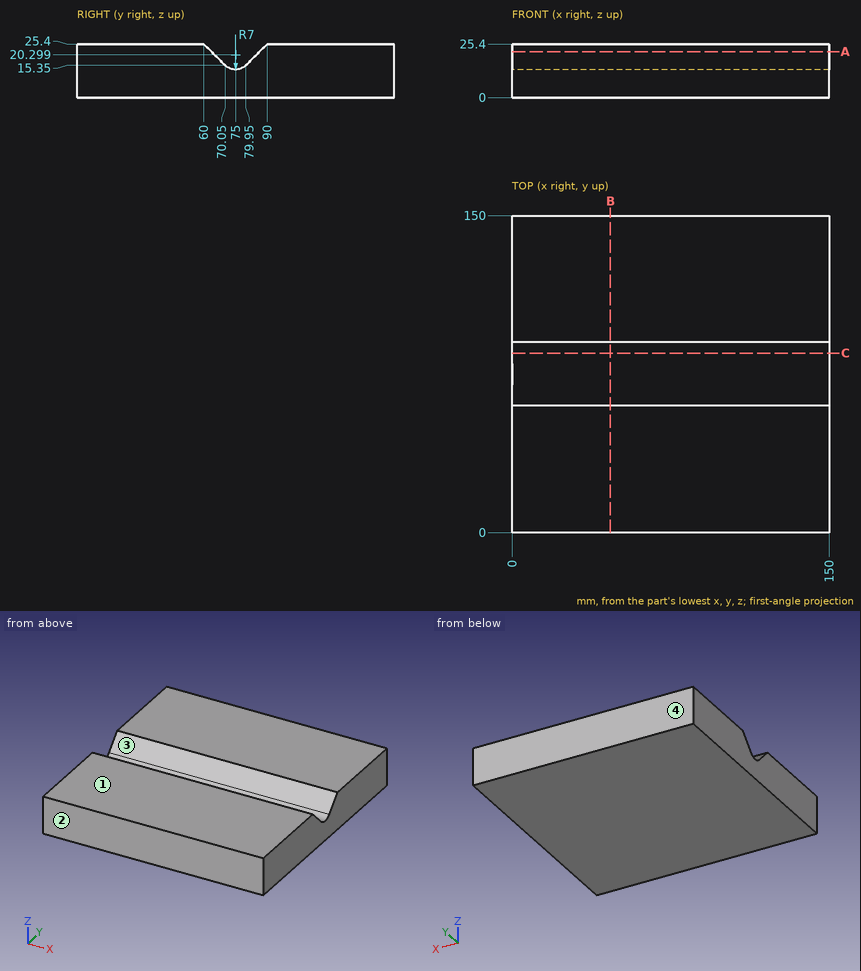
Geometry: see drawing. Coordinates: mm, zero at the bounding-box minimum. Give positions to 0.01 mm unless a question says otherwise; leave off trailing zeros. Order: outer loops, then holes, each group sorted by start corner. A loop starts at its lowest first (then second) coordinate and runs counter-clockwise, first axis right, second up.
Q1. Draft query along Y for the marked faces 1, 2, 3 and 4. Return one class per face: +Y half, -Y half, draft (parallel to the pull), parting line (faces both ways), or undercut.
Checked values:
face 1: draft
face 2: -Y half
face 3: undercut
face 4: +Y half
Q2. Section B-B on x = 46.5. Output: boundary loops of the cut face in (y, z), and give its area (3 significant figures).
Checked values:
outline: (0, 0) - (150, 0) - (150, 25.4) - (90, 25.4) - (79.95, 15.35) arc R7 cw to (70.05, 15.35) - (60, 25.4) - (0, 25.4) - close
area: 3,600 mm2
Q3. Section C-C on y = 85. Output: boundary loops of the cut face in (x, z).
Checked values:
outline: (0, 0) - (150, 0) - (150, 20.4) - (0, 20.4) - close
Q4. Ray query, probe 1 along Y at (x, z) = (84.5, 22.5); probe 2 along Y at (x, z) = (60, 18.75). Return the intervals inside material, ascending.
Checked values:
probe 1: y = 0 to 62.9, 87.1 to 150
probe 2: y = 0 to 66.65, 83.35 to 150
Q5. Section A-A on z = 21.75. Output: boundary loops of the cut face in (x, y), and give its area (3 significant figures).
Checked values:
outline: (0, 0) - (150, 0) - (150, 63.65) - (0, 63.65) - close; (0, 86.35) - (150, 86.35) - (150, 150) - (0, 150) - close
area: 19,100 mm2
Q6. Contact query for flat-ended pins moving along their axis: pin 1 Ø8 at (y, z) = (34, 9) entering from -X; pin 2 Ø1.5 at (x, y) = (60.5, 67.5) entering from +Z. Output: stop coordinate, or through.
Checked values:
pin 1: stops at x = 0
pin 2: stops at z = 18.65
